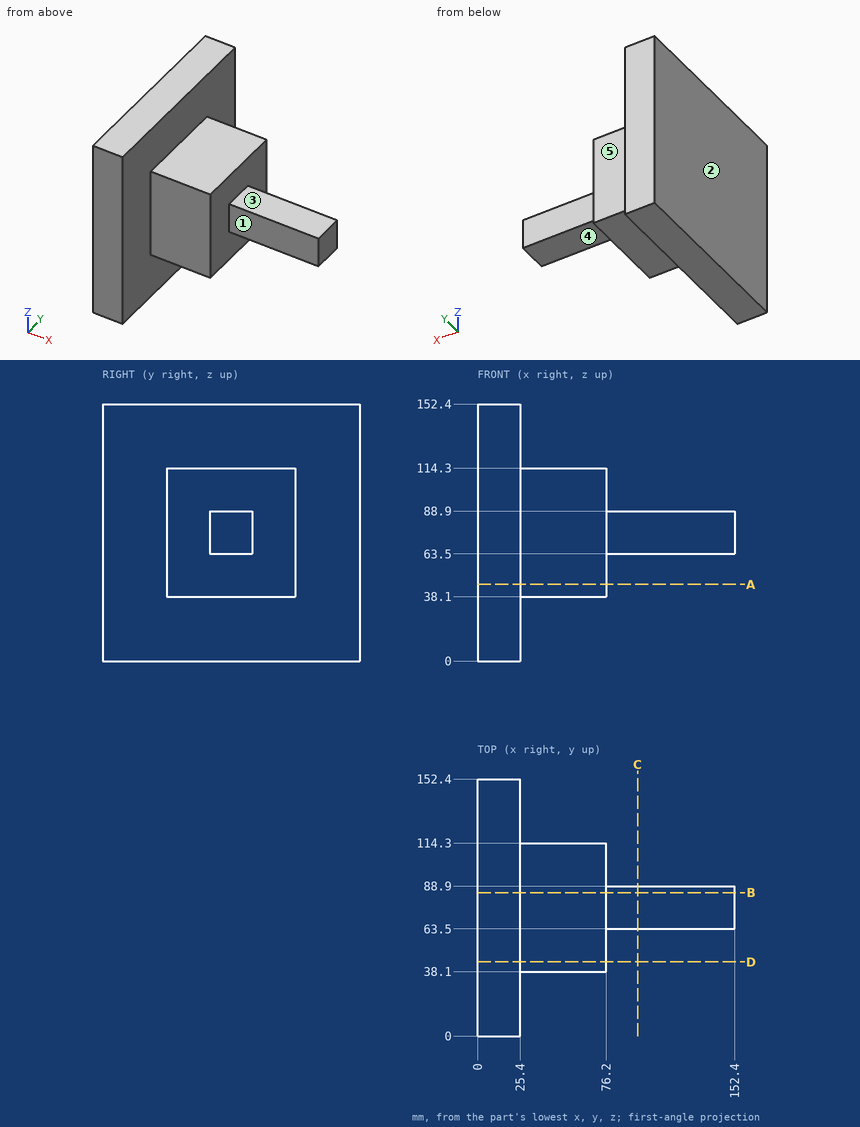
Could you check a few things on this drawing? It's one solid part, dimensions in mm from its lowest x, y, z. A direction names the side the tool comes from. Give positions to 0.01 mm unless a question says otherwise; leave off trailing zeros. Order: outer loops, then holes, each group sorted by start corner. A loop starts at its lowest first (then second) coordinate and runs counter-clockwise, first axis right, second up. Notation, with made-up numbers: (-34, 51.5) -> (-25, 51.5) arc R24 cw to (-25, 89.5) -> close; hole circle Ø1 at (-38, 30). An arc over 180 degrees is marked (long way). Answer in a Markdown table with one row per item. Add a question column.
Item 1: For the marked faces 1, 2, 3, 4 and 5, which set-ups out of +Z, -Z, +X, -X, +Y, -Y let a thin tool reach every point of the face, with its end or its side?
Item 2: I'm going to push flat-ended pins straight in: P1, Ø23, axis at y = 63, z = 94.5, coming from the +X side; P2, Ø15, axis at x = 47, y = 86, coming from the -Z side; P3, Ø10, axis at y = 37.5, z = 88, coming from the +X side; P4, Ø1.5, axis at x = 76, z = 115, coming from the +Y side. Where does each tip first touch, or does it pass through?
Item 3: Please list where these lines run through material, in increasing order: probe 1 along Z at (x, y) = (72.5, 54); probe 2 along X at (y, z) = (25, 60.5); probe 3 along X at (y, z) = (105, 86).
Item 4: Imagine slicing it at A-A (z = 45.5). List the corners of the cut face in (x, y) for me, and give its area (3 significant figures).
Item 5: Imagine slicing it at C-C (x = 95). List the corners of the cut face in (y, z) for me, and give its area (3 significant figures).
Item 6: Imagine slicing it at B-B (y = 85). List the corners of the cut face in (x, z) for me.
Result:
| question | item | result |
|---|---|---|
| 1 | face 1 | +Z, -Z, +X, -Y |
| 1 | face 2 | +Z, -Z, -X, +Y, -Y |
| 1 | face 3 | +Z, +X, +Y, -Y |
| 1 | face 4 | -Z, +X, +Y, -Y |
| 1 | face 5 | +Z, -Z, +X, +Y |
| 2 | P1 | x = 152.4 |
| 2 | P2 | z = 38.1 |
| 2 | P3 | x = 76.2 |
| 2 | P4 | y = 114.3 |
| 3 | probe 1 | 38.1 to 114.3 |
| 3 | probe 2 | 0 to 25.4 |
| 3 | probe 3 | 0 to 76.2 |
| 4 | outline | (0, 0) -> (25.4, 0) -> (25.4, 38.1) -> (76.2, 38.1) -> (76.2, 114.3) -> (25.4, 114.3) -> (25.4, 152.4) -> (0, 152.4) -> close |
| 4 | area | 7,740 mm2 |
| 5 | outline | (63.5, 63.5) -> (88.9, 63.5) -> (88.9, 88.9) -> (63.5, 88.9) -> close |
| 5 | area | 645 mm2 |
| 6 | outline | (0, 0) -> (25.4, 0) -> (25.4, 38.1) -> (76.2, 38.1) -> (76.2, 63.5) -> (152.4, 63.5) -> (152.4, 88.9) -> (76.2, 88.9) -> (76.2, 114.3) -> (25.4, 114.3) -> (25.4, 152.4) -> (0, 152.4) -> close |
